```python
from build123d import *

# Parameters (mm, degrees)
SKETCH1_W            = 150
SKETCH1_H            = 105
SKETCH1_R            = 8.75
SKETCH1_R_2          = 2.75
BASE_DEPTH           = 6.35
SKETCH3_R            = 4.9
SKETCH3_R_2          = 1.65
BEARING_HOLES_DEPTH  = 7.35
SKETCH2_R            = 1.65
MOUNTING_HOLES_DEPTH = 7.35


with BuildPart() as part:
    # Sketch1 → Base (new body)
    with BuildSketch(Plane(origin=(0, 0, 0), x_dir=(1, 0, 0), z_dir=(0, 1, 0))):
        Rectangle(SKETCH1_W, SKETCH1_H)
        Circle(SKETCH1_R, mode=Mode.SUBTRACT)
        with Locations((10.102788136, 10.102788136)):
            Circle(SKETCH1_R_2, mode=Mode.SUBTRACT)
        with Locations((10.102788136, -10.102788136)):
            Circle(SKETCH1_R_2, mode=Mode.SUBTRACT)
        with Locations((-10.102788136, -10.102788136)):
            Circle(SKETCH1_R_2, mode=Mode.SUBTRACT)
        with Locations((-10.102788136, 10.102788136)):
            Circle(SKETCH1_R_2, mode=Mode.SUBTRACT)
    extrude(amount=BASE_DEPTH)

    # Sketch3 → Bearing Holes (cut, through all)
    with BuildSketch(Plane(origin=(0, 6.35, 0), x_dir=(1, 0, 0), z_dir=(0, 1, 0))):
        with Locations((37.5, 0)):
            Circle(SKETCH3_R)
        with Locations((26.3875, 11.1125)):
            Circle(SKETCH3_R_2)
        with Locations((48.6125, 11.1125)):
            Circle(SKETCH3_R_2)
        with Locations((48.6125, -11.1125)):
            Circle(SKETCH3_R_2)
        with Locations((26.3875, -11.1125)):
            Circle(SKETCH3_R_2)
        with Locations((-26.3875, -11.1125)):
            Circle(SKETCH3_R_2)
        with Locations((-48.6125, -11.1125)):
            Circle(SKETCH3_R_2)
        with Locations((-48.6125, 11.1125)):
            Circle(SKETCH3_R_2)
        with Locations((-26.3875, 11.1125)):
            Circle(SKETCH3_R_2)
        with Locations((-37.5, 0)):
            Circle(SKETCH3_R)
    extrude(amount=-BEARING_HOLES_DEPTH, mode=Mode.SUBTRACT)

    # Sketch2 → Mounting Holes (cut, through all)
    with BuildSketch(Plane(origin=(0, 6.35, 0), x_dir=(1, 0, 0), z_dir=(0, 1, 0))):
        with Locations((-65, 37.5)):
            Circle(SKETCH2_R)
        with Locations((-65, -37.5)):
            Circle(SKETCH2_R)
        with Locations((65, -37.5)):
            Circle(SKETCH2_R)
        with Locations((65, 37.5)):
            Circle(SKETCH2_R)
    extrude(amount=-MOUNTING_HOLES_DEPTH, mode=Mode.SUBTRACT)


solid = part.part
```
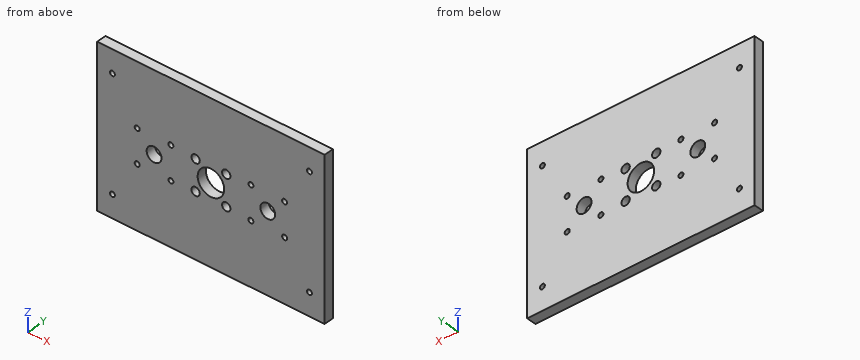
Could you check a few things on this model? Use its own coordinates, in mm. Coordinates: 2 decimals unless noted, no trailing zeros. Order: outer loops, then holes, each group sorted by start corner. A loop starts at its lowest first (then second) coordinate and runs counter-clockwise, first axis right, second up. Notation, with made-up numbers: M 20.25,31 L 55.25,31 A28 ccw 55.25,69 Z; hole C 77.5,43.25 d8. An arc over 180 degrees is marked long. Use a Markdown table: item, result. Add a question column.
Q1. I want a section at B-B on z = -37.5. List the corners of the cut face in (x, y) for me, then the cut area to 3 significant figures.
Q2. If I drill on L1, parallel to Z at x = -65, y = 2.25; L2, parallel to Z at x = 0, y = 1.75; L3, parallel to Z at x = 38, y = 6, over which ranges is the centre line in solid material (lowest first)?
Q3. I want a section at A-A on x = -65. List the corners of the cut face in (y, z) for me, then the cut area to 3 significant figures.
Q4. I want a section at D-D on y = 2. Give the number of separate pieces and of enclosed holes in the cut face, then the cut area to 3 significant figures.
Q5. I want a section at C-C on x = 37.5. List the corners of the cut face in (y, z) for me.
Checked values:
| question | item | result |
|---|---|---|
| 1 | outline | M -75,0 L -66.65,0 L -66.65,6.35 L -75,6.35 Z; M -63.35,0 L 63.35,0 L 63.35,6.35 L -63.35,6.35 Z; M 66.65,0 L 75,0 L 75,6.35 L 66.65,6.35 Z |
| 1 | area | 911 mm² |
| 2 | L1 | -52.5 to -39.15, -35.85 to 35.85, 39.15 to 52.5 |
| 2 | L2 | -52.5 to -8.75, 8.75 to 52.5 |
| 2 | L3 | -52.5 to -4.87, 4.87 to 52.5 |
| 3 | outline | M 0,-52.5 L 6.35,-52.5 L 6.35,-39.15 L 0,-39.15 Z; M 0,-35.85 L 6.35,-35.85 L 6.35,35.85 L 0,35.85 Z; M 0,39.15 L 6.35,39.15 L 6.35,52.5 L 0,52.5 Z |
| 3 | area | 625 mm² |
| 4 | separate pieces | 1 |
| 4 | enclosed holes | 19 |
| 4 | area | 15,200 mm² |
| 5 | outline | M 0,-52.5 L 6.35,-52.5 L 6.35,-4.9 L 0,-4.9 Z; M 0,4.9 L 6.35,4.9 L 6.35,52.5 L 0,52.5 Z |
